```python
from build123d import *

# Parameters (mm, degrees)
BOSS_EXTRUDE1_START     = -114.3
BOSS_EXTRUDE1_OUTLINE_R = 3.175
BOSS_EXTRUDE1_DEPTH     = 114.3


# Read off the part's stored shape, not the designer's step: Boss-Extrude1
with BuildPart() as part:
    # Boss-Extrude1 outline → Boss-Extrude1 (new body)
    with BuildSketch(Plane.XY.offset(98.3791731).offset(BOSS_EXTRUDE1_START)):
        Circle(BOSS_EXTRUDE1_OUTLINE_R)
    extrude(amount=BOSS_EXTRUDE1_DEPTH)


solid = part.part
```
Could you check a few things on this model? Use its own coordinates, in mm. Coordinates: 2 decimals unless noted, no trailing zeros. Order: outer loops, then holes, each group sorted by start corner. A loop starts at its lowest first (then second) coordinate and runs counter-clockwise, first axis right, second up. Notation, with made-up numbers: M 71.5,66 L 116.5,66 A11 ccw 116.5,87 Z; hole C 14.25,82.25 d3. An arc over 180 degrees is marked long. Use a Markdown table: item, result. Add a question column.
Q1. I want a section at B-B on y = -1. List the corners of the cut face in (x, z) for me.
Q2. If I drill on L1, parallel to Y at x = -0.25, z = 18.5; L2, parallel to Y at x = 1.5, z = 41.5, over which ranges is the centre line in solid material (lowest first)?
Q3. I want a section at A-A on z = 64.5. List the corners of the cut face in (x, y) for me (3 decimals).
Q4. I'm going to push flat-ended pins straight in: pin 1 (1.5 mm diameter, centred on y = 1.5, z = 10, fed in from -X); pin 2 (1 mm diameter, centred on x = -1, z = 4, fed in from +Y). Where does each tip first touch, or does it pass through?
Q5. I want a section at C-C on x = -1.5. List the corners of the cut face in (y, z) for me.
Checked values:
| question | item | result |
|---|---|---|
| 1 | outline | M -3.01,-15.92 L 3.01,-15.92 L 3.01,98.38 L -3.01,98.38 Z |
| 2 | L1 | -3.17 to 3.17 |
| 2 | L2 | -2.8 to 2.8 |
| 3 | outline | C 0,0 d6.35 |
| 4 | pin 1 | x = -3.09 |
| 4 | pin 2 | y = 3.14 |
| 5 | outline | M -2.8,-15.92 L 2.8,-15.92 L 2.8,98.38 L -2.8,98.38 Z |
